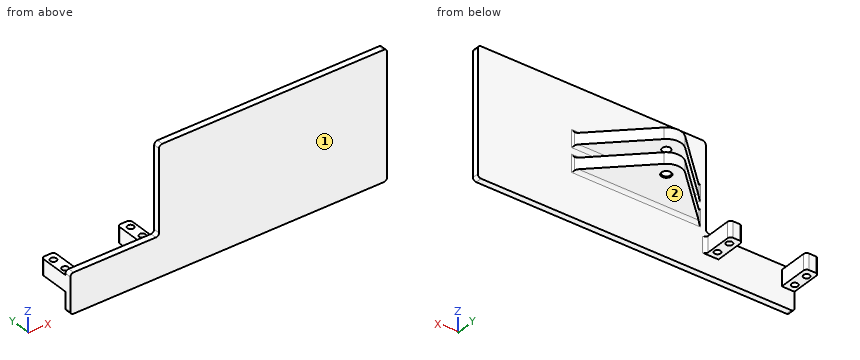
```python
from build123d import *

# Parameters (mm, degrees)
SKETCH1_R           = 2.6
BOSS_EXTRUDE1_DEPTH = 22
SKETCH2_W           = 200
SKETCH2_H           = 80
BOSS_EXTRUDE2_DEPTH = 4
SKETCH3_W           = 8
SKETCH3_H           = 35
CUT_EXTRUDE1_DEPTH  = 209.42744541
CHAMFER1_SIZE       = 0.5
BOSS_EXTRUDE3_START = -22
SKETCH4_W           = 8
SKETCH4_H           = 20
SKETCH4_R           = 2
BOSS_EXTRUDE3_DEPTH = 10
SKETCH5_W           = 56
SKETCH5_H           = 55
CUT_EXTRUDE2_DEPTH  = 7
FILLET1_R           = 2


with BuildPart() as part:
    # Sketch1 → Boss-Extrude1 (new body)
    with BuildSketch(Plane.XY):
        with BuildLine():
            Line((-6.63831163, 6.934898608), (-40, -25))
            Line((-40, -25), (40, -25))
            Line((40, -25), (6.63831163, 6.934898608))
            ThreePointArc((6.63831163, 6.934898608), (0, 9.6), (-6.63831163, 6.934898608))
        make_face()
        Circle(SKETCH1_R, mode=Mode.SUBTRACT)
    extrude(amount=BOSS_EXTRUDE1_DEPTH)

    # Sketch2 → Boss-Extrude2 (add)
    with BuildSketch(Plane(origin=(0, -25, 0), x_dir=(-1, 0, 0), z_dir=(0, -1, 0))):
        with Locations((0, -11)):
            Rectangle(SKETCH2_W, SKETCH2_H)
    extrude(amount=BOSS_EXTRUDE2_DEPTH)

    # Sketch3 → Cut-Extrude1 (cut, through all)
    with BuildSketch(Plane(origin=(100, 0, 0), x_dir=(0, 0, -1), z_dir=(1, 0, 0))):
        with Locations((-11, -7.5)):
            Rectangle(SKETCH3_W, SKETCH3_H)
    extrude(amount=-CUT_EXTRUDE1_DEPTH, mode=Mode.SUBTRACT)

    # Chamfer1
    chamfer1_edges = [part.edges().sort_by_distance(p)[0] for p in [
        (-2.6, 0, 0),
        (-2.6, 0, 22),
    ]]
    chamfer(chamfer1_edges, length=CHAMFER1_SIZE)

    # Sketch4 → Boss-Extrude3 (add)
    # profile 1 of 2: a face of its own
    with BuildSketch(Plane(origin=(0, 0, -29), x_dir=(-1, 0, 0), z_dir=(0, 0, -1)).offset(BOSS_EXTRUDE3_START)):
        with Locations((96, -15)):
            Rectangle(SKETCH4_W, SKETCH4_H)
        with Locations((96.4, -20)):
            Circle(SKETCH4_R, mode=Mode.SUBTRACT)
        with Locations((96.4, -10.2)):
            Circle(SKETCH4_R, mode=Mode.SUBTRACT)
    # profile 2 of 2: a face of its own
    with BuildSketch(Plane(origin=(0, 0, -29), x_dir=(-1, 0, 0), z_dir=(0, 0, -1)).offset(BOSS_EXTRUDE3_START)):
        with Locations((48, -15)):
            Rectangle(SKETCH4_W, SKETCH4_H)
        with Locations(Location((47.6, -20, 0), (0, 0, 180))):
            Circle(SKETCH4_R, mode=Mode.SUBTRACT)
        with Locations(Location((47.6, -10.2, 0), (0, 0, 180))):
            Circle(SKETCH4_R, mode=Mode.SUBTRACT)
    extrude(amount=BOSS_EXTRUDE3_DEPTH)

    # Sketch5 → Cut-Extrude2 (cut)
    with BuildSketch(Plane(origin=(0, -25, 0), x_dir=(1, 0, 0), z_dir=(0, 1, 0))):
        with Locations((-72, -23.5)):
            Rectangle(SKETCH5_W, SKETCH5_H)
    extrude(amount=-CUT_EXTRUDE2_DEPTH, mode=Mode.SUBTRACT)

    # Fillet1
    fillet1_edges = [part.edges().sort_by_distance(p)[0] for p in [
        (-100, -5, -12),
        (-92, -5, -12),
        (-44, -5, -12),
        (-52, -5, -12),
        (-44, -25, -12),
        (0, -25, 0),
        (0, -25, 15),
        (-40, -25, 18.5),
        (0, -25, 7),
        (-40, -25, 3.5),
        (0, -25, 22),
        (40, -25, 3.5),
        (40, -25, 18.5),
        (100, -27, -29),
        (100, -27, 51),
        (-100, -27, -29),
        (-44, -27, -4),
        (-44, -27, 51),
        (-100, -27, -4),
    ]]
    fillet(fillet1_edges, radius=FILLET1_R)


solid = part.part
```
The model under review builds one solid part; all positions refer to its coordinate system, in mm. Face numbers are marked on the shaded views. A direction names the side the tool comes from. Round coordinates to 2 decimals unless told otherwise and drop trailing zeros. Order: outer loops, then holes, each group sorted by start corner. A loop starts at its lowest first (then second) coordinate and runs counter-clockwise, first axis right, second up. Notation, with made-up numbers: (15.25, -4) -> (47.25, -4) arc R13 cw to (47.25, 20) -> close; hole circle Ø9 at (-40, 35). An arc over 180 degrees is marked (long way). One line per item, written item: value. Start each with the question number.
Q1. Take a section at A-A (z = -10.5). Write out the cut boundary in (x, y).
Q2. Take a section at D-D (y = 0). Write out the cut boundary in (x, z), and give its area (3 significant figures).
Q3. Wall thickness on line 1 (Y direction, x = -47.6, z = -9.5); line 2 (X direction, y = -10, z = -13); line 3 (Z direction, x = 3, y = -7): over which ranges is each line inside the solid? List them lowest first.
Q4. Take a section at C-C (y = -20). Write out the cut boundary in (x, z).
Q5. Machinability: for the marked faces 1 and 2, which of the approach directions +Z, -Z, +X, -X, +Y, -Y give a long, thin tool a straight path to every point of the face, cutting with its end or side? Answer none if there is none.
Q6. Clearance check with flat-ended pins moving along their axes: pin 1 Ø8 at (y, z) = (5.5, 23.5) entering from +X; pin 2 Ø8 at (y, z) = (-9, -6) entering from +X; pin 3 Ø1.2 at (x, y) = (-71, -27) entering from +Z. State where each tip first meets the part, or that it passes through.
Q7. Take a section at B-B (x = 0). Write out the cut boundary in (y, z), and give its area (3 significant figures).
Reported:
1. outline: (-100, -29) -> (100, -29) -> (100, -25) -> (-42, -25) arc R2 cw to (-44, -23) -> (-44, -7) arc R2 ccw to (-46, -5) -> (-50, -5) arc R2 ccw to (-52, -7) -> (-52, -25) -> (-92, -25) -> (-92, -7) arc R2 ccw to (-94, -5) -> (-98, -5) arc R2 ccw to (-100, -7) -> close; hole circle Ø4 at (-96.4, -20); hole circle Ø4 at (-96.4, -10.2); hole circle Ø4 at (-47.6, -20); hole circle Ø4 at (-47.6, -10.2)
2. outline: (-13.88, 0) -> (-3.1, 0) -> (-2.6, 0.5) -> (-2.6, 7) -> (-13.88, 7) -> close; (-13.88, 15) -> (-2.6, 15) -> (-2.6, 21.5) -> (-3.1, 22) -> (-13.88, 22) -> close; (2.6, 0.5) -> (3.1, 0) -> (13.88, 0) -> (13.88, 7) -> (2.6, 7) -> close; (2.6, 15) -> (13.88, 15) -> (13.88, 22) -> (3.1, 22) -> (2.6, 21.5) -> close
2. area: 315 mm2
3. line 1: y = -29 to -22, -18 to -12.2, -8.2 to -5
3. line 2: x = -100 to -98.39, -94.41 to -92, -52 to -49.59, -45.61 to -44
3. line 3: z = 0 to 7, 15 to 22
4. outline: (-100, -17) -> (-98.4, -17) -> (-98.4, -7) -> (-100, -7) -> close; (-94.4, -17) -> (-92, -17) -> (-92, -7) -> (-94.4, -7) -> close; (-52, -17) -> (-49.6, -17) -> (-49.6, -7) -> (-52, -7) -> close; (-45.6, -17) -> (-44, -17) -> (-44, -7) -> (-45.6, -7) -> close; (-34.78, 0) -> (34.78, 0) -> (34.78, 7) -> (-34.78, 7) -> close; (-34.78, 15) -> (34.78, 15) -> (34.78, 22) -> (-34.78, 22) -> close
5. face 1: +Z, -Z, +X, -X, -Y
5. face 2: -Z, +X, -X, +Y
6. pin 1: stops at x = 12.01
6. pin 2: stops at x = -44
6. pin 3: stops at z = -4
7. outline: (-29, -29) -> (-25, -29) -> (-25, -2) arc R2 cw to (-23, 0) -> (-3.1, 0) -> (-2.6, 0.5) -> (-2.6, 7) -> (-23, 7) arc R2 cw to (-25, 9) -> (-25, 13) arc R2 cw to (-23, 15) -> (-2.6, 15) -> (-2.6, 21.5) -> (-3.1, 22) -> (-23, 22) arc R2 cw to (-25, 24) -> (-25, 51) -> (-29, 51) -> close; (2.6, 0.5) -> (3.1, 0) -> (9.6, 0) -> (9.6, 7) -> (2.6, 7) -> close; (2.6, 15) -> (9.6, 15) -> (9.6, 22) -> (3.1, 22) -> (2.6, 21.5) -> close
7. area: 735 mm2
